Geometry: final body of the model. Coordinates: model frame, mm. A direction names the side the tool comes from. Give positions to 0.01 mm unless a question says otherwise; leave off trailing zeros. Order: outer loops, then holes, each group sorted by start corner. A loop starts at its lowest first (then second) coordinate and runs counter-clockwise, first axis right, second up. Notation, with made-up numbers: (2, -7) - (59, -7) arc R25 ccw to (59, 10) - close; hole circle Ø7 at (39.25, 47). An arc over 180 degrees is marked (long way). Put each result on its own line as item: value. Start each with the question number.
1. Ray query, line 1 along Y through (x, z) = (0, 0.8); line 2 along Y through (x, z) = (0, 1); line 3 along Z through (x, y) = (4, -6.75). Return the intervals inside material, ascending. Write a range as from..to.
2. Section B-B on z = 3.05. Return the cut outline in (x, y), plus the area to 3 significant figures.
3. Mould query, pull axis X, two halves, no side actions, for faces 4 (the flat face through (2, -2, 0)), 5 (the conical face through (7.243, 2.281, 2.656)), 6 (the flat face through (0, 0, 2)). Classes: pulls with the +X half, pulls with the -X half, needs draft (parallel to the pull), parting line crosses it, or undercut.
4. Set-up query: faces 1 (the conical face through (7.243, -2.281, 2.344)), 2 (the flat face through (0, 0, 5)), 3 (the cylindrical face through (0.54, -2.44, 0.99)). Return all of +Z, -Z, +X, -X, +Y, -Y with unobstructed straight access to the full face (end or side cutting, diameter ignored); none if empty.
5. First-contact query: P1, Ø1.5, axis at x = -5.5, y = 3, coming from the -Z side; P2, Ø1.5, axis at y = -2.5, z = 2, coming from the -X side; P3, Ø2, axis at y = -5.5, z = 3, coming from the -X side; P4, Ø1.5, axis at x = 1, y = -0.5, coming from the -Z side. Flat tips, straight axial feed; report the tip coordinate or a pass-through.
6. Section A-A on x = 0. Return the cut outline in (y, z).
Autodesk Inventor part; units mm, degrees
ref_plane "작업 평면2" through (0, 0, 2.5) normal (0, 0, 1) x (1, 0, 0)
ref_plane "작업 평면1" through (0, 0, 5) normal (0, 0, 1) x (1, 0, 0)
ref_plane "YZ Plane" through (0, 0, 0) normal (1, 0, 0) x (0, 1, 0)
sketch "스케치1" plane through (0, 0, 0) normal (0, 0, 1) x (1, 0, 0)
  circle A0 centre (0, 0) radius 9
  dimension "d0" = 18
ref_plane "작업 평면2" through (0, 0, 2.5) normal (0, 0, 1) x (1, 0, 0)
sketch "스케치2" plane through (0, 0, 2.5) normal (0, 0, 1) x (1, 0, 0)
  circle A0 centre (0, 0) radius 7.5
  dimension "d3" = 15
ref_plane "작업 평면1" through (0, 0, 5) normal (0, 0, 1) x (1, 0, 0)
sketch "스케치3" plane through (0, 0, 5) normal (0, 0, 1) x (1, 0, 0)
  circle A0 centre (0, 0) radius 9
loft "로프트1" add profiles "스케치3", "스케치2"
loft "로프트2" add profiles "스케치1" section 2 edges at (-7.5, 0, 2.5)
sketch "스케치4" plane through (0, 0, 0) normal (0, 0, -1) x (-1, 0, 0)
  circle A0 centre (0, 0) radius 2.5
  dimension "d13" = 5
extrude "돌출2" cut sketch "스케치4" against normal blind 2
properties part number "wheel"
Resolved:
1. line 1: -8.52..-2.5, 2.5..8.52
1. line 2: -8.4..-2.5, 2.5..8.4
1. line 3: 0..1.92, 3.08..5
2. outline: circle Ø15.66 at (0, 0)
2. area: 193 mm^2
3. face 4: needs draft
3. face 5: parting line crosses it
3. face 6: undercut
4. face 1: none
4. face 2: +Z, +X, -X, +Y, -Y
4. face 3: -Z
5. P1: z = 0
5. P2: x = -7.91
5. P3: x = -6.68
5. P4: z = 2
6. outline: (-9, 0) - (-2.5, 0) - (-2.5, 2) - (2.5, 2) - (2.5, 0) - (9, 0) - (7.5, 2.5) - (9, 5) - (-9, 5) - (-7.5, 2.5) - close
